Study the drawing (mm; zero at the part's minimum x, y, z) and answer. Coordinates: 2 decimals unless noted, no trailing zeros. Order: outer loops, then holes, each group sorted by start corner. A loop starts at its lowest first (then second) coordinate and runs counter-clockwise, first axis right, second up. Notation, with made-up numbers: (69, 5) - (121, 5) arc R18 ccw to (121, 37) - close; hole circle Ø4 at (-14.75, 86). An arc over 180 degrees is marked (long way). Write item = value, one per line.
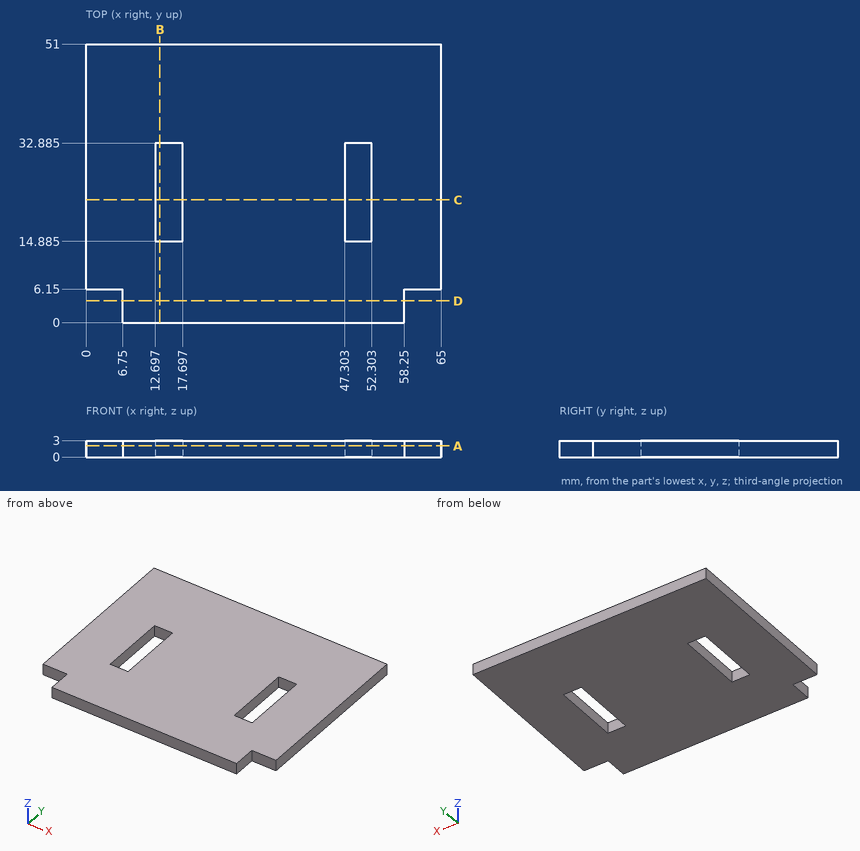
1) A flat-ended cylindrical pin translates along its axis: pin 1 Ø1.5 at (y, z) = (3.5, 1) entering from +X. Find the tip coordinate at first contact, or state that the pin passes through.
Returned:
pin_1 = 58.25
2) Straight lines are drawn through the part: line 1 along X through (y, z) = (20, 0.9); line 2 along Y through (x, z) = (47.5, 2.9) (1 decimal); line 3 along Y through (x, z) = (59, 2.35). For each, find the intervals that lie inside material, in ascending order. Write a range as from..to.
Returned:
line_1 = 0..12.7, 17.7..47.3, 52.3..65
line_2 = 0..14.9, 32.9..51
line_3 = 6.15..51
3) The part is cut by section C-C (y = 22.5). Determine the outline of the cut face in (x, z), and give its area (3 significant figures).
Returned:
outline = (0, 0) - (12.7, 0) - (12.7, 3) - (0, 3) - close; (17.7, 0) - (47.3, 0) - (47.3, 3) - (17.7, 3) - close; (52.3, 0) - (65, 0) - (65, 3) - (52.3, 3) - close
area = 165 mm^2
4) The part is cut by section A-A (z = 2.05). Count the separate pieces of the cut face and the enclosed holes in it, and give its area (3 significant figures).
Returned:
separate_pieces = 1
enclosed_holes = 2
area = 3,050 mm^2
5) The part is cut by section B-B (x = 13.5). Determine the outline of the cut face in (y, z) (1 decimal).
Returned:
outline = (0, 0) - (14.9, 0) - (14.9, 3) - (0, 3) - close; (32.9, 0) - (51, 0) - (51, 3) - (32.9, 3) - close
6) The part is cut by section D-D (y = 4). Determine the outline of the cut face in (x, z).
Returned:
outline = (6.75, 0) - (58.25, 0) - (58.25, 3) - (6.75, 3) - close
